Source: three-view drawing plus pictorial views. Frame: mm from the lowest corner of the part. Round coordinates to 2 decimals unless told otherwise and drop trailing zeros. Answer as CSV lines item,"result". Start each with the question number.
1) Section query A-A, the plane y = 1.5. State how many separate pieces and enclosed holes the cut face has, and give its area (3 significant figures).
2) First-contact query: P1, Ø3, axis at y = 5, z = 17.5, coming from the -X side. Flat tip, straight axial feed; report the tip coordinate or a pass-through.
3) Line query: L1, parallel to X at y = 4.75, z = 12; L2, parallel to Z at x = 871, y = 1.5. Output: solid intervals per line, ascending.
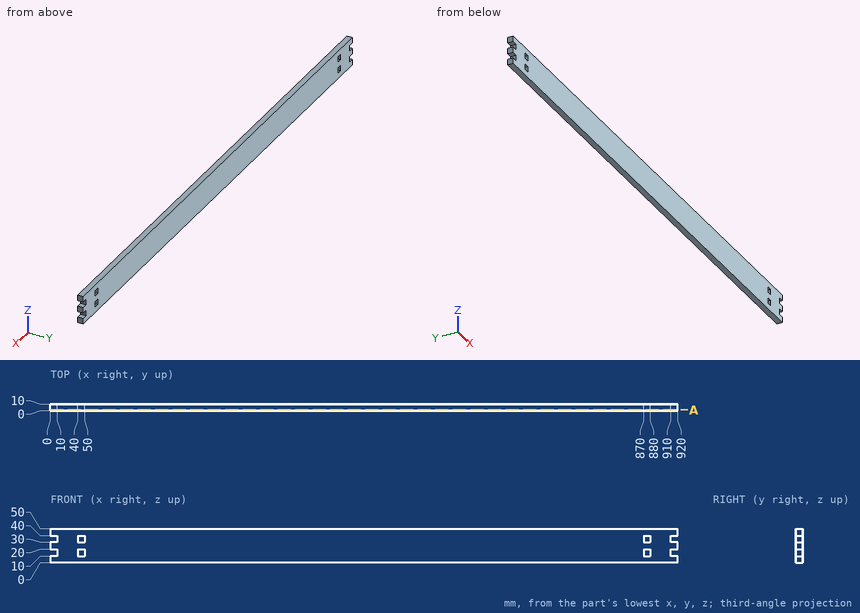
Findings:
1,separate pieces,"1"
1,enclosed holes,"4"
1,area,"45,200 mm^2"
2,P1,"stops at x = 10"
3,L1,"x = 10 to 40, 50 to 870, 880 to 910"
3,L2,"z = 0 to 10, 20 to 30, 40 to 50"
